```python
from build123d import *

# Parameters (mm, degrees)
SKETCH1_R           = 1
BOSS_EXTRUDE1_DEPTH = 1.6
SKETCH2_W           = 5
SKETCH2_H           = 4
BOSS_EXTRUDE2_DEPTH = 1.5


with BuildPart() as part:
    # Sketch1 → Boss-Extrude1 (new body)
    with BuildSketch(Plane.XY):
        with BuildLine():
            Line((-5.678908346, -7), (5.678908346, -7))
            ThreePointArc((5.678908346, -7), (6.664901072, -6.068697859), (7.5, -5))
            Line((7.5, -5), (7.5, 5))
            ThreePointArc((7.5, 5), (0, 9.013878189), (-7.5, 5))
            Line((-7.5, 5), (-7.5, -5))
            ThreePointArc((-7.5, -5), (-6.664901072, -6.068697859), (-5.678908346, -7))
        make_face()
        with Locations((-6, 0)):
            Circle(SKETCH1_R, mode=Mode.SUBTRACT)
        with Locations((6, 0)):
            Circle(SKETCH1_R, mode=Mode.SUBTRACT)
    extrude(amount=BOSS_EXTRUDE1_DEPTH)

    # Sketch2 → Boss-Extrude2 (add)
    with BuildSketch(Plane.XY.offset(1.6)):
        Rectangle(SKETCH2_W, SKETCH2_H)
    extrude(amount=BOSS_EXTRUDE2_DEPTH)


solid = part.part
```
Read the model definition and answer for the solid it produces. Units are mm, in the model's axes. A direction names the side the tool comes from. Round coordinates to 2 decimals unless told otherwise and drop trailing zeros. Write each loop counter-clockwise with the first axis right and the second up, starting at its lowest first coordinate (ties: lowest second). Pieces come first, ordered by that corner, then holes. Notation, with made-up numbers: (-25, 5) -> (-20, 5) arc R24 ccw to (-20, 36) -> close; hole circle Ø8 at (-0.5, -3). An arc over 180 degrees is marked (long way). Answer in a Markdown table with one row per item. Add a question column.
1) Find section A-A, the plane y = 0. Determine the outline of the cut face in (x, z), and give its area (3 significant figures).
2) Find section C-C, the plane z = 0.55. Determine the outline of the cut face in (x, y), and give its area (3 significant figures).
3) Which of the six approach directions +Z, -Z, +X, -X, +Y, -Y give full straight-line access (tool end or side, diameter ignored) to faces 1 (the face through (0, -2, 2)), 2 (the face through (0, 1, 0)), 3 (the face through (-2.5, 0, 2)), 4 (the face through (2.5, 0, 2)), 5 (the face through (0, 2, 2))?
4) Consider line 1 (Y direction, x = 6, z = 0.6); line 2 (X direction, y = -0.5, z = 2.3); line 3 (Z direction, x = 6.75, y = -3.5). Determine where each line is inside the solid, lowest interval first.
5) Determine the mould class of faces 6 (the face through (0.124, 9.013, 0.789)), 7 (the face through (5.2, -0.6, 0.8)), 8 (the face through (-7.5, 0, 1)) for opening direction Y: pulls with the +Y half, pulls with the -Y half, needs draft (parallel to the pull), parting line crosses it, or undercut.
6) Find section B-B, the plane x = -6. Determine the outline of the cut face in (y, z), and give its area (3 significant figures).
7) Find section D-D, the plane x = -0.5. Determine the outline of the cut face in (y, z), and give its area (3 significant figures).
8) Given P1, Ø1.6, axis at x = 6, y = 0, coming from the +Z side; P2, Ø0.8, axis at x = 0.5, z = 2.5, coming from the +Y side; P3, Ø3, axis at x = -6, y = 0, coming from the +Z side; P4, Ø1, axis at y = 6, z = 1.5, coming from the -X side, each flat-ended and moving along its own axis, determine where each tip first touches the part or whether it passes through.
Findings below:
| question | item | result |
|---|---|---|
| 1 | outline | (-7.5, 0) -> (-7, 0) -> (-7, 1.6) -> (-7.5, 1.6) -> close; (-5, 0) -> (5, 0) -> (5, 1.6) -> (2.5, 1.6) -> (2.5, 3.1) -> (-2.5, 3.1) -> (-2.5, 1.6) -> (-5, 1.6) -> close; (7, 0) -> (7.5, 0) -> (7.5, 1.6) -> (7, 1.6) -> close |
| 1 | area | 25.1 mm² |
| 2 | outline | (-7.5, -5) arc R9.01 ccw to (-5.68, -7) -> (5.68, -7) arc R9.01 ccw to (7.5, -5) -> (7.5, 5) arc R9.01 ccw to (-7.5, 5) -> close; hole circle Ø2 at (-6, 0); hole circle Ø2 at (6, 0) |
| 2 | area | 213 mm² |
| 3 | face 1 | +Z, +X, -X, -Y |
| 3 | face 2 | -Z, +X, -X, +Y, -Y |
| 3 | face 3 | +Z, -X, +Y, -Y |
| 3 | face 4 | +Z, +X, +Y, -Y |
| 3 | face 5 | +Z, +X, -X, +Y |
| 4 | line 1 | -6.73 to -1, 1 to 6.73 |
| 4 | line 2 | -2.5 to 2.5 |
| 4 | line 3 | 0 to 1.6 |
| 5 | face 6 | pulls with the +Y half |
| 5 | face 7 | undercut |
| 5 | face 8 | needs draft |
| 6 | outline | (-6.73, 0) -> (-1, 0) -> (-1, 1.6) -> (-6.73, 1.6) -> close; (1, 0) -> (6.73, 0) -> (6.73, 1.6) -> (1, 1.6) -> close |
| 6 | area | 18.3 mm² |
| 7 | outline | (-7, 0) -> (9, 0) -> (9, 1.6) -> (2, 1.6) -> (2, 3.1) -> (-2, 3.1) -> (-2, 1.6) -> (-7, 1.6) -> close |
| 7 | area | 31.6 mm² |
| 8 | P1 | through |
| 8 | P2 | y = 2 |
| 8 | P3 | z = 1.6 |
| 8 | P4 | x = -7.14 |
